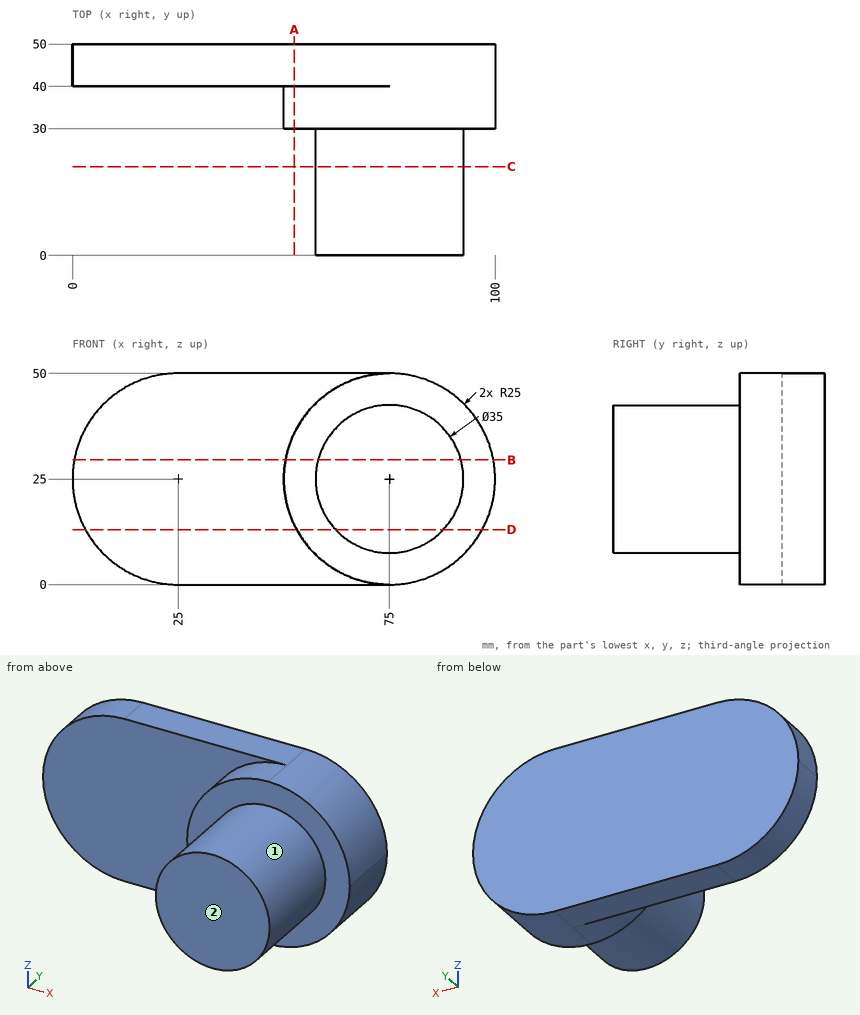
Can you work these out from the drawing? Everything is in mm from the part's minimum corner. A direction names the side the tool comes from. Coordinates: 2 decimals unless noted, no trailing zeros. Loops run counter-clockwise (first coordinate to the right, second up) from the corner with the lowest first, then second, coordinate; pieces in that order, holes last.
1. Imagine slicing it at B-B, the plane z = 29.5. Please give me the cut outline in (x, y).
2. Imagine slicing it at A-A, the plane x = 52.5. Please give me the cut outline in (y, z), and give its area (3 significant figures).
3. I need wall thicknesses on L1, parallel to Y at x = 94.5, z = 23; L2, parallel to Y at x = 5.5, z = 23.5; L3, parallel to X at y = 24.5, z = 10.5. Which ranges of each line are inside material? Lowest first, please.
4. Imagine slicing it at C-C, the plane y = 21. Please give me the cut outline in (x, z), and give its area (3 significant figures).
5. For the marked faces 1 and 2, which set-ups out of +Z, -Z, +X, -X, +Y, -Y let a thin tool reach every point of the face, with its end or its side?
6. For P1, Ø8, axis at y = 21.5, z = 5, coming from the +X side; P2, Ø6, axis at y = 9.5, z = 37, coming from the -X side; P3, Ø2, axis at y = 32.5, z = 16.5, coming from the +X side, each with a flat end and sliding along its axis, tell me the tip position at first contact or that it passes through.
7. Imagine slicing it at D-D, the plane z = 13. Please give me the cut outline in (x, y).
Taken from the geometry:
1. outline: (0.41, 40) - (50.41, 40) - (50.41, 30) - (58.09, 30) - (58.09, 0) - (91.91, 0) - (91.91, 30) - (99.59, 30) - (99.59, 50) - (0.41, 50) - close
2. outline: (30, 14.1) - (40, 14.1) - (40, 0) - (50, 0) - (50, 50) - (40, 50) - (40, 35.9) - (30, 35.9) - close
2. area: 718 mm2
3. L1: y = 30 to 50
3. L2: y = 40 to 50
3. L3: x = 65.2 to 84.8
4. outline: circle Ø35 at (75, 25)
4. area: 962 mm2
5. face 1: -Y
5. face 2: +Z, -Z, +X, -X, -Y
6. P1: stops at x = 82.09
6. P2: stops at x = 59.99
6. P3: stops at x = 98.85
7. outline: (3.07, 40) - (53.07, 40) - (53.07, 30) - (62.26, 30) - (62.26, 0) - (87.74, 0) - (87.74, 30) - (96.93, 30) - (96.93, 50) - (3.07, 50) - close
